```python
from build123d import *

# Parameters (mm, degrees)
EXTRUDE_THIN2_DEPTH      = 180.34
EXTRUDE_THIN2_DEPTH_BACK = 2.54
FILLET1_R                = 2.54
FILLET2_R                = 2.54
FILLET3_R                = 2.54
FILLET4_R                = 2.54
FILLET5_R                = 2.54
FILLET6_R                = 2.54
FILLET7_R                = 2.54


with BuildPart() as part:
    # Sketch2 → Extrude-Thin2 (new, two sides: drawn at the far end of the back side and taken through both)
    with BuildSketch(Plane.XY.offset(-EXTRUDE_THIN2_DEPTH_BACK)):
        Polygon((-12.274730593, 5.817033739), (-9.228474815, 5.817033739), (-9.228474815, 0), (15.619605828, 0), (15.619605828, 5.848528279), (18.694831425, 5.848528279), (18.694831425, 8.388528279), (13.079605828, 8.388528279), (13.079605828, 2.54), (-6.688474815, 2.54), (-6.688474815, 8.357033739), (-12.274730593, 8.357033739), align=None)
    extrude(amount=EXTRUDE_THIN2_DEPTH + EXTRUDE_THIN2_DEPTH_BACK)

    # Fillet1
    fillet1_edges = [part.edges().sort_by_distance(p)[0] for p in [
        (-6.688474815, 2.54, 88.9),
        (13.079605828, 2.54, 88.9),
        (13.079605828, 5.46426414, 180.34),
        (3.195565506, 2.54, 180.34),
        (-6.688474815, 5.44851687, 180.34),
        (13.079605828, 5.46426414, -2.54),
        (3.195565506, 2.54, -2.54),
        (-6.688474815, 5.44851687, -2.54),
    ]]
    fillet(fillet1_edges, radius=FILLET1_R - 0.0001)  # a hair under: the kernel refuses the full size

    # Fillet2
    fillet2_edges = [part.edges().sort_by_distance(p)[0] for p in [
        (15.619605828, 5.848528279, 88.9),
    ]]
    fillet(fillet2_edges, radius=FILLET2_R)

    # Fillet3
    fillet3_edges = [part.edges().sort_by_distance(p)[0] for p in [
        (17.157168626, 8.388528279, -2.54),
        (17.157168626, 8.388528279, 180.34),
        (13.079605828, 8.388528279, 88.9),
        (13.823525314, 8.388528279, 179.596080514),
        (13.823525314, 8.388528279, -1.796080514),
    ]]
    fillet(fillet3_edges, radius=FILLET3_R - 0.0001)  # a hair under: the kernel refuses the full size

    # Fillet4
    fillet4_edges = [part.edges().sort_by_distance(p)[0] for p in [
        (15.619605828, 0, 88.9),
    ]]
    fillet(fillet4_edges, radius=FILLET4_R)

    # Fillet5
    fillet5_edges = [part.edges().sort_by_distance(p)[0] for p in [
        (-10.751552704, 8.357033739, -2.54),
        (-6.688474815, 8.357033739, 88.9),
        (-10.751552704, 8.357033739, 180.34),
        (-7.432394301, 8.357033739, 179.596080514),
        (-7.432394301, 8.357033739, -1.796080514),
    ]]
    fillet(fillet5_edges, radius=FILLET5_R - 0.0001)  # a hair under: the kernel refuses the full size

    # Fillet6
    fillet6_edges = [part.edges().sort_by_distance(p)[0] for p in [
        (-9.228474815, 0, 88.9),
    ]]
    fillet(fillet6_edges, radius=FILLET6_R)

    # Fillet7
    fillet7_edges = [part.edges().sort_by_distance(p)[0] for p in [
        (-9.228474815, 5.817033739, 88.9),
    ]]
    fillet(fillet7_edges, radius=FILLET7_R)


solid = part.part
```
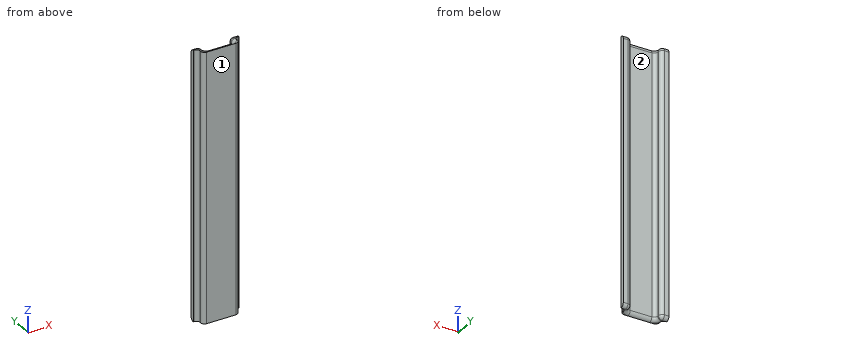
The listing builds one solid part. Answer for the finished solid, in the listing's coordinates (mm). Face numbers are marked on the shaded views. Give positions to 0.01 mm unless a question says otherwise; leave off trailing zeros. Order: outer loops, then holes, each group sorted by start corner. A loop starts at its lowest first (then second) coordinate and runs counter-clockwise, first axis right, second up. Notation, with made-up numbers: (41.5, 10.25) -> (73.5, 10.25) arc R14 cw to (73.5, 19.25) -> close; hole circle Ø11 at (84.5, -4). An arc over 180 degrees is marked (long way). One line per item, written item: value.
1) Determine the mould class of the marked faces 1 and 2 for opening direction X: pulls with the +X half, pulls with the -X half, needs draft (parallel to the pull), parting line crosses it, or undercut.
Reported:
face 1: needs draft
face 2: undercut
2) Flat-ended cylindrical pins translate along their axes: P1, Ø1.5, axis at x = 6.5, z = 73, coming from the +Y side; P2, Ø3, axis at y = 1.5, z = 63.5, coming from the -X side; P3, Ø1.5, axis at x = -11, z = 86, coming from the +Y side. Find the tip coordinate at first contact, or state that the pin passes through.
Reported:
P1: stops at y = 2.54
P2: stops at x = -9.23
P3: stops at y = 8.36
3) Find the intervals of material crossed by line 1 (Y direction, x = -6, z = 74); line 2 (Y direction, x = 4, z = 75); line 3 (X direction, y = 6.5, z = 99), in increasing order.
Reported:
line 1: y = 0 to 3.34
line 2: y = 0 to 2.54
line 3: x = -12.27 to -6.78, 13.16 to 18.69
4) Find section B-B, the plane z = 23. Determine the outline of the cut face in (x, y).
Reported:
outline: (-12.27, 5.82) -> (-11.77, 5.82) arc R2.54 cw to (-9.23, 3.28) -> (-9.23, 2.54) arc R2.54 ccw to (-6.69, 0) -> (13.08, 0) arc R2.54 ccw to (15.62, 2.54) -> (15.62, 3.31) arc R2.54 cw to (18.16, 5.85) -> (18.69, 5.85) -> (18.69, 8.39) -> (15.62, 8.39) arc R2.54 ccw to (13.08, 5.85) -> (13.08, 5.08) arc R2.54 cw to (10.54, 2.54) -> (-4.15, 2.54) arc R2.54 cw to (-6.69, 5.08) -> (-6.69, 5.82) arc R2.54 ccw to (-9.23, 8.36) -> (-12.27, 8.36) -> close
